Design review of the part built by this model. Coordinates are the model's own, in mm. Face numbers are marked on the shaded views. A direction names the side the tool comes from. Coordinates: 2 decimals unless noted, no trailing zeros. Loops run counter-clockwise (first coordinate to the right, second up) from the corner with the lowest first, then second, coordinate; pieces in that order, holes last. Notation, with made-up numbers: (83, 16) - (115, 16) arc R23 ccw to (115, 55) - close; hole circle Ø4 at (-40, 28). An arc over 180 degrees is marked (long way). Use one line per item in the form item = value. Start each with the question number.
(1) For L1, parallel to Y at x = 4, z = 1.75; L2, parallel to Y at x = -1, z = 7; L3, parallel to Z at x = 0, y = 8.7, list the stretches that pass through material, from the lowest coordinate up.
(2) Clearance check with flat-ended pins moving along their axes: pin 1 Ø2 at (x, z) = (0, 5) entering from +Y; pin 2 Ø3 at (y, z) = (10, 7) entering from -X; pin 3 Ø1 at (x, z) = (11.5, 1.5) entering from -Y. State where each tip first meets the part, or that it passes through.
(3) Add section A-A (x = 0). State the section outline as (y, z) points, plus the area to 3 significant figures.
(4) Add section C-C (y = 4.25). Count the separate pieces of the cut face and the enclosed holes in it, plus the area to 3 significant figures.
(5) Add section B-B (z = 1.25). State the section outline as (x, y) points, plus the area to 3 significant figures.
(6) Tool access review of the marked faces 4, 5, 6, 7 and 8: name each direction out of +Z, -Z, +X, -X, +Y, -Y from which nothing blocks a thin tool from reaching the whole face with its end or side.
(7) The part is to be moulded in two halves that separate along Y. For the marked faces 1, 2 and 3, say which applies: pulls with the +Y half, pulls with the -Y half, needs draft (parallel to the pull), parting line crosses it, or undercut.
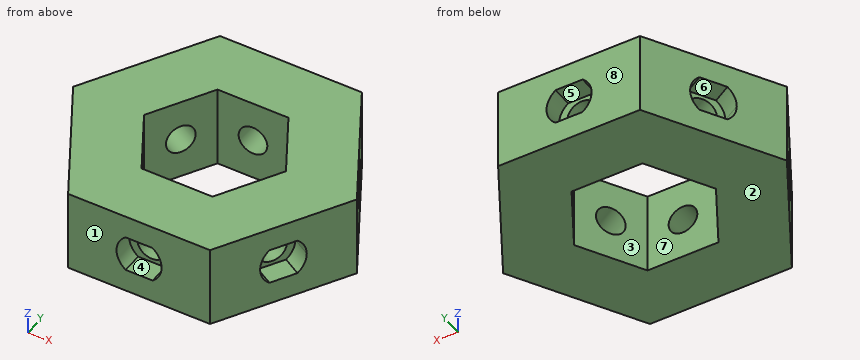
```python
from build123d import *

# Parameters (mm, degrees)
F1_DEPTH = 10
F2_R     = 1.75
F3_DEPTH = 25
F4_DEPTH = 2.5
F6_COUNT = 6
F8_DEPTH = 25


with BuildPart() as f1:
    # F0 (on Top) → F1 (new body)
    with BuildSketch(Plane.XY):
        Polygon((-8.660254, -15), (8.660254, -15), (0, 0), align=None)
    extrude(amount=F1_DEPTH)

    # F2 (on face) → F3 (cut)
    with BuildSketch(Plane.XZ.offset(15)):
        with Locations((0, 5)):
            Circle(F2_R)
    extrude(amount=-F3_DEPTH, mode=Mode.SUBTRACT)

    # F2 (on face) → F4 (cut)
    with BuildSketch(Plane.XZ.offset(15)):
        with BuildLine():
            ThreePointArc((1.65, 2.8), (2.459675, 3.770163), (2.75, 5))
            ThreePointArc((2.75, 5), (2.459675, 6.229837), (1.65, 7.2))
            Line((1.65, 7.2), (-1.65, 7.2))
            ThreePointArc((-1.65, 7.2), (-2.75, 5), (-1.65, 2.8))
            Line((-1.65, 2.8), (1.65, 2.8))
        make_face()
        with Locations((0, 5)):
            Circle(F2_R, mode=Mode.SUBTRACT)
    extrude(amount=-F4_DEPTH, mode=Mode.SUBTRACT)

    # F6: F1 ×6 about axis
    f6_axis = Axis((0, 0, 7.747169), (0, 0, 1))


with BuildPart() as f1_1:
    add(f1.part)
    for i in range(1, F6_COUNT):
        add(f1.part.rotate(f6_axis, i * 360 / F6_COUNT))

    # F7 (on face) → F8 (cut)
    with BuildSketch(Plane.XY.offset(10)):
        Polygon((-4.330127, -7.5), (4.330127, -7.5), (8.660254, 0), (4.330127, 7.5), (-4.330127, 7.5), (-8.660254, 0), align=None)
    extrude(amount=-F8_DEPTH, mode=Mode.SUBTRACT)


solid = f1_1.part
```
Computed values:
q1.L1 = -15 to -7.5, 7.5 to 15
q1.L2 = -12.5 to -7.5, 7.5 to 12.5
q1.L3 = 0 to 3.25, 6.75 to 10
q2.pin_1 = through
q2.pin_2 = -12.41
q2.pin_3 = -10.95
q3.outline = (-15, 0) - (-7.5, 0) - (-7.5, 3.25) - (-12.5, 3.25) - (-12.5, 2.8) - (-15, 2.8) - close; (-15, 7.2) - (-12.5, 7.2) - (-12.5, 6.75) - (-7.5, 6.75) - (-7.5, 10) - (-15, 10) - close; (7.5, 0) - (15, 0) - (15, 2.8) - (12.5, 2.8) - (12.5, 3.25) - (7.5, 3.25) - close; (7.5, 6.75) - (12.5, 6.75) - (12.5, 7.2) - (15, 7.2) - (15, 10) - (7.5, 10) - close
q3.area = 93.0 mm^2
q4.separate_pieces = 2
q4.enclosed_holes = 2
q4.area = 142 mm^2
q5.outline = (-17.32, 0) - (-8.66, -15) - (8.66, -15) - (17.32, 0) - (8.66, 15) - (-8.66, 15) - close; hole (-8.66, 0) - (-4.33, -7.5) - (4.33, -7.5) - (8.66, 0) - (4.33, 7.5) - (-4.33, 7.5) - close
q5.area = 585 mm^2
q6.face_4 = -Y
q6.face_5 = +Y
q6.face_6 = none
q6.face_7 = +Z, -Z
q6.face_8 = +Z, -Z, +X, -X, +Y
q7.face_1 = pulls with the -Y half
q7.face_2 = needs draft
q7.face_3 = undercut
